```python
from build123d import *

# Parameters (mm, degrees)
F0_W     = 8
F0_H     = 4.6
F2_R     = 5.5
F2_R_2   = 2
F3_DEPTH = 0.3
F4_W     = 5.5
F4_H     = 11.2
F6_R     = 2
F7_DEPTH = 3.9


with BuildPart() as f1:
    # F0 (on Front) → F1 (revolve)
    with BuildSketch(Plane.XZ):
        with Locations((6, 0.039412)):
            Rectangle(F0_W, F0_H)
    revolve(axis=Axis((0, 0, 0.039412), (0, 0, -1)))

    # F2 (on face) → F3 (join)
    with BuildSketch(Plane.XY.offset(2.339412)):
        Circle(F2_R)
        Circle(F2_R_2, mode=Mode.SUBTRACT)
    extrude(amount=F3_DEPTH)


with BuildPart() as f5:
    # F4 (on Front) → F5 (revolve)
    with BuildSketch(Plane.XZ):
        with Locations((2.75, 8.252153)):
            Rectangle(F4_W, F4_H)
    revolve(axis=Axis((0, 0, 8.252153), (0, 0, 1)))

    # F6 (on face) → F7 (join)
    with BuildSketch(Plane.XY.offset(13.852153)):
        Circle(F6_R)
    extrude(amount=F7_DEPTH)


with BuildPart() as f9:
    # F8 (on Front) → F9 (revolve)
    with BuildSketch(Plane.XZ):
        Polygon((2, 17.76988), (0, 17.76988), (0, 2.691046), (2, 2.691046), (2, -2.23012), (10, -2.23012), (10, 2.66988), (5.491101, 2.66988), (5.491101, 13.86988), (2, 13.86988), align=None)
    revolve(axis=Axis((0, 0, 4.709774), (0, 0, -1)))


solid = f9.part
```
For this review, take the finished solid that the model builds, in its own axes (mm). A direction names the side the tool comes from. Coordinates: 2 decimals unless noted, no trailing zeros. Loops run counter-clockwise (first coordinate to the right, second up) from the corner with the lowest first, then second, coordinate; pieces in that order, holes last. Notation, with made-up numbers: (11.5, 34.5) -> (62.5, 34.5) arc R20 ccw to (62.5, 55.5) -> close; hole circle Ø9 at (-35, 74). An arc over 180 degrees is marked (long way). Return JSON: item names as keys, results as strings. Group by question number.
(1) To check wall thickness, follow L1, parallel to Y at x = 0, z = 0.35; L2, parallel to Y at x = 0.75, z = 0. State the ranges of each line that lie inside material, in increasing order.
(2) Mouldability with a two-part tool opening along X and no side actions: class faces 1 (the cylindrical face through (0, 2, 0)), 2 (the cylindrical face through (5.238, -1.649, 8.348)), 3 (the flat face through (4, 4, 2.67)) as pulls with the +X half, pulls with the -X half, needs draft (parallel to the pull), parting line crosses it, or undercut.
(3) Consider section C-C, the plane z = 8.5. Give the boundary of the cut face in (x, y).
(4) Consider section A-A, the plane y = 0. Give the boundary of the cut face in (x, z).
(5) Tool access review of faces 4 (the flat face through (2.4, -0.1, 13.87)), 5 (the flat face through (0, 0, 17.77)), 6 (the flat face through (0, 0, 2.691)): name each direction out of +Z, -Z, +X, -X, +Y, -Y from which nothing blocks a thin tool from reaching the whole face with its end or side.
(6) Consider section D-D, the plane z = 1.5. Give the boundary of the cut face in (x, y), plus the area to 3 significant figures.
(7) For pin 1 Ø10 at (y, z) = (1, 14.5) entering from -X; pin 2 Ø1.5 at (x, z) = (2.5, 12) entering from +Y; pin 3 Ø4 at (y, z) = (2, 3.5) entering from -X, all flat-tipped, find the tip position at first contact; note any pin that passes through.
Results below:
{
 "1": {"L1": "y = -10 to -2, 2 to 10", "L2": "y = -9.97 to -1.85, 1.85 to 9.97"},
 "2": {"face 1": "undercut", "face 2": "parting line crosses it", "face 3": "needs draft"},
 "3": {"outline": "circle Ø10.98 at (0, 0)"},
 "4": {"outline": "(-10, -2.23) -> (-2, -2.23) -> (-2, 2.69) -> (2, 2.69) -> (2, -2.23) -> (10, -2.23) -> (10, 2.67) -> (5.49, 2.67) -> (5.49, 13.87) -> (2, 13.87) -> (2, 17.77) -> (-2, 17.77) -> (-2, 13.87) -> (-5.49, 13.87) -> (-5.49, 2.67) -> (-10, 2.67) -> close"},
 "5": {"face 4": "+Z", "face 5": "+Z, +X, -X, +Y, -Y", "face 6": "-Z"},
 "6": {"outline": "circle Ø20 at (0, 0); hole circle Ø4 at (0, 0)", "area": "302 mm2"},
 "7": {"pin 1": "stops at x = -5.49", "pin 2": "stops at y = 5.2", "pin 3": "stops at x = -10"}
}
